Autodesk Inventor part; units mm, degrees
ref_plane "Начальная плоскость" through (0, 0, 0) normal (0, 0, 1) x (1, 0, 0)
ref_plane "Конечная плоскость" through (0, 0, 1) normal (0, 0, 1) x (1, 0, 0)
ref_plane "YZ Plane" through (0, 0, 0) normal (1, 0, 0) x (0, 1, 0)
ref_plane "Начальная плоскость" through (0, 0, 0) normal (0, 0, 1) x (1, 0, 0)
ref_plane "Конечная плоскость" through (0, 0, 1) normal (0, 0, 1) x (1, 0, 0)
sketch "Эскиз" plane through (0, 0, 0) normal (0, 0, 1) x (1, 0, 0)
  line L0 (-1.2, -2.1) -> (-1.2, 15.2)
  line L1 (-4.2, 16.4) -> (-2.4, 16.4)
  line L2 (-4.2, -8.6) -> (-4.2, 16.4)
  line L3 (-4.2, -8.6) -> (11.8, -8.6)
  line L4 (11.8, -6.8) -> (11.8, -8.6)
  line L5 (2.3, -5.6) -> (10.6, -5.6)
  arc A0 (-1.2, -2.1) -> (2.3, -5.6) centre (2.3, -2.1) ccw
  arc A1 (-1.2, 15.2) -> (-2.4, 16.4) centre (-2.4, 15.2) ccw
  arc A2 (11.8, -6.8) -> (10.6, -5.6) centre (10.6, -6.8) ccw
  line L6 (11.8, 0) -> (-4.2, 0) construction
  line L7 (0, -8.6) -> (0, 16.4) construction
  line L8 (0, 0) -> (16, 0) construction
  point P0 (-1.2, -5.6)
  point P1 (-1.2, 16.4)
  point P2 (11.8, -5.6)
  dimension "d17" = 3.5
  dimension "d19" = 1.2
  dimension "d26" = 8.6
  dimension "d27" = 4.2
  dimension "d28" = 25
  dimension "d29" = 16
  dimension "d30" = 3
  dimension "d31" = 3
  dimension "d32" = 90
extrude "Базовый элемент" add sketch "Эскиз" along normal up to surface (1 mm away) from surface at 0
sketch "Sketch3" plane through (0, 0, 0) normal (0, 0, 1) x (1, 0, 0)
  line L0 (0, 0) -> (10, 0)
ref_plane "Work Plane10" through (0, 0, 0) normal (0, -1, 0) x (1, 0, 0)
sketch "Sketch4" plane through (0, 0, 0) normal (0, -1, 0) x (1, 0, 0)
  line L0 (-2, 0) -> (12, 0)
  line L1 (-2, 1) -> (12, 1)
  dimension "d25" = 1
equation "\"d17\" = R"
equation "\"d19\" = r1"
equation "\"d26\" = ey"
equation "\"d27\" = ex"
equation "\"d28\" = b"
equation "\"d29\" = a"
equation "\"d30\" = ParT"
equation "\"d31\" = ParT"
equation "\"d11\" = G_L"
equation "\"b\" = 25"
equation "\"ParT\" = 3"
equation "\"R\" = 3.5"
equation "\"G_L\" = d25"
equation "\"r1\" = 1.2"
equation "\"G_OFFSET_START\" = 0"
equation "\"G_OFFSET_END\" = 0"
equation "\"d21\" = G_OFFSET_END + B_L"
equation "\"ex\" = 4.2"
equation "\"ey\" = 8.6"
equation "\"B_L\" = 1"
equation "\"a\" = 16"
properties part number "Кутик ДСТУ 2251" material "С245 ДСТУ 8539"
Geometry check sheet. Reference: the model listing, model coordinates, mm. A direction names the side the tool comes from. Give positions to 0.01 mm unless a question says otherwise; leave off trailing zeros. Write each loop counter-clockwise with the first axis right and the second up, starting at its lowest first coordinate (ties: lowest second). Pieces come first, ordered by that corner, then holes. Notation, with made-up numbers: M 4.5,83.5 L 23.5,83.5 A13 cw 23.5,90.5 Z; hole C -35.5,45.25 d8. An arc over 180 degrees is marked long. Answer as CSV lines item,"result". Start each with the question number.
Q1. Material ranges on L1, parallel to Y at x = 4.5, z = 0.95; L2, parallel to X at y = 14.75, z = 0.3; L3, parallel to Y at x = -1.5, z = 0.75, recorded low to high.
Q2. Tool access check on faces 1 (the face through (-3.3, 16.4, 0.5)), 2 (the face through (-1.2, 6.4, 0.5)). Record the directions out of +Z, -Z, +X, -X, +Y, -Y that give a thin tool (end or side, any length) a straight path to the whole face; none if there is none.
Q3. Go/stop test with a flat-tipped pin: pin 1 (0.5 mm diameter, centred on x = 4.5, z = 0.5, fed in from +Y). Record where the tip stops, or that it passes through.
Q4. Section check B-B, the plane y = 0.5. Record the cut outline in (x, z), then the cut area to 3 significant figures.
Q5. Section check A-A, the plane z = 0.5. Record the cut outline in (x, y).
Q6. Section check C-C, the plane x = 7. Record the cut outline in (y, z), then the cut area to 3 significant figures.
Geometry says:
1,L1,"-8.6 to -5.6"
1,L2,"-4.2 to -1.2"
1,L3,"-8.6 to 15.99"
2,face 1,"+Z, -Z, +X, -X, +Y"
2,face 2,"+Z, -Z, +X, +Y"
3,pin 1,"y = -5.6"
4,outline,"M -4.2,0 L -1.2,0 L -1.2,1 L -4.2,1 Z"
4,area,"3.00 mm^2"
5,outline,"M -4.2,-8.6 L 11.8,-8.6 L 11.8,-6.8 A1.2 ccw 10.6,-5.6 L 2.3,-5.6 A3.5 cw -1.2,-2.1 L -1.2,15.2 A1.2 ccw -2.4,16.4 L -4.2,16.4 Z"
6,outline,"M -8.6,0 L -5.6,0 L -5.6,1 L -8.6,1 Z"
6,area,"3.00 mm^2"
